Source: three-view drawing plus pictorial views. Frame: mm from the lowest corner of the part. A direction names the side the tool comes from. Give positions to 0.01 mm unless a question says otherwise; leave off trailing zeros. Write each loop counter-clockwise with the first axis right and the second up, starting at its lowest first coordinate (ties: lowest second). Pieces come first, ordered by that corner, then holes. Notation, with made-up numbers: (-14, 65.5) -> (35, 65.5) arc R23 cw to (35, 77.5) -> close; hole circle Ø10 at (-29.75, -23). An arc over 180 degrees is marked (long way). Answer in a Markdown table with one row per item. Add a question column.
Item 1: Section query D-D on z = 1.5. Output: boundary loops of the cut face in (x, y).
Item 2: Section query C-C on y = 16.5. Output: boundary loops of the cut face in (x, z), plus the area to 3 significant figures.
Item 3: Material intervals for probe 1 along X at (y, z) = (14.75, 5); probe 2 along X at (y, z) = (10.5, 5); probe 3 along Z at (x, y) = (77, 18.5), sorted ascending. Write a range as from..to.
Item 4: Section query B-B on z = 5. Output: boundary loops of the cut face in (x, y).
Item 5: Draft query along X for the marked faces 3, 4, 5 and 6. Return one class per face: +X half, -X half, draft (parallel to the pull), parting line (faces both ways), or undercut.
Item 6: First-contact query: P1, Ø1.5, axis at x = 57.5, z = 3, coming from the -Y side. Flat tip, straight axial feed; report the tip coordinate or a pass-through.
Item 7: Access query for the marked faces 1 and 2. Directions: +Z, -Z, +X, -X, +Y, -Y. A direction counts if a zero-diameter tool reaches every point of the face in a straight line with its end or side. Return the directions, or none.
Item 8: Section query A-A on x = 5. Output: boundary loops of the cut face in (y, z).
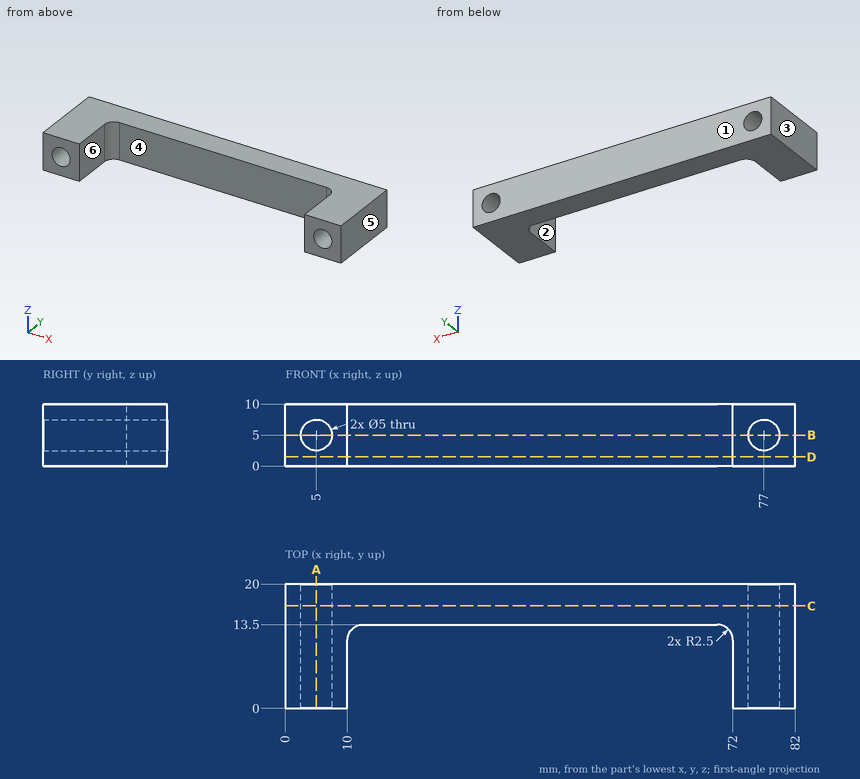
Findings below:
| question | item | result |
|---|---|---|
| 1 | outline | (0, 0) -> (10, 0) -> (10, 11) arc R2.5 cw to (12.5, 13.5) -> (69.5, 13.5) arc R2.5 cw to (72, 11) -> (72, 0) -> (82, 0) -> (82, 20) -> (0, 20) -> close |
| 2 | outline | (0, 0) -> (82, 0) -> (82, 10) -> (0, 10) -> close; hole circle Ø5 at (5, 5); hole circle Ø5 at (77, 5) |
| 2 | area | 781 mm^2 |
| 3 | probe 1 | x = 0..2.5, 7.5..74.5, 79.5..82 |
| 3 | probe 2 | x = 0..2.5, 7.5..10, 72..74.5, 79.5..82 |
| 3 | probe 3 | z = 0..2.5, 7.5..10 |
| 4 | outline | (0, 0) -> (2.5, 0) -> (2.5, 20) -> (0, 20) -> close; (7.5, 0) -> (10, 0) -> (10, 11) arc R2.5 cw to (12.5, 13.5) -> (69.5, 13.5) arc R2.5 cw to (72, 11) -> (72, 0) -> (74.5, 0) -> (74.5, 20) -> (7.5, 20) -> close; (79.5, 0) -> (82, 0) -> (82, 20) -> (79.5, 20) -> close |
| 5 | face 3 | -X half |
| 5 | face 4 | undercut |
| 5 | face 5 | +X half |
| 5 | face 6 | undercut |
| 6 | P1 | stops at y = 13.5 |
| 7 | face 1 | +Z, -Z, +X, -X, +Y |
| 7 | face 2 | +Z, -Z, -Y |
| 8 | outline | (0, 0) -> (20, 0) -> (20, 2.5) -> (0, 2.5) -> close; (0, 7.5) -> (20, 7.5) -> (20, 10) -> (0, 10) -> close |
